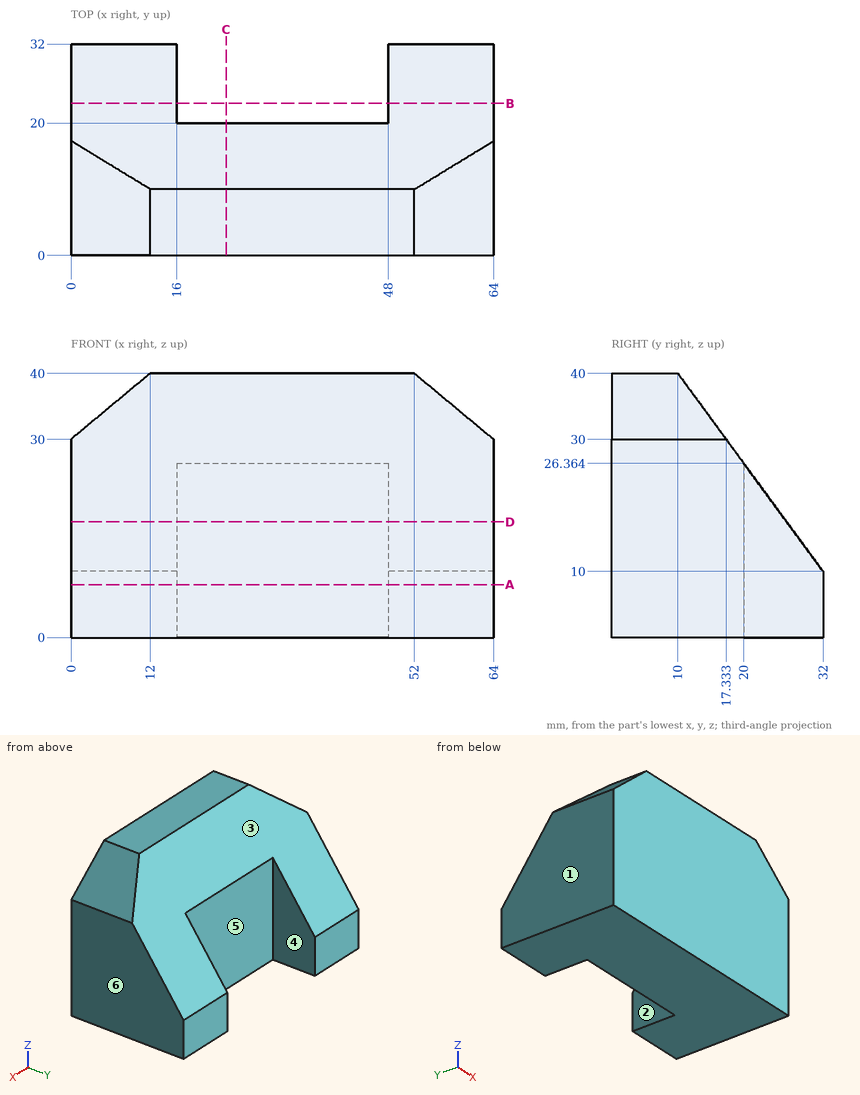
Study the drawing (mm; zero at the part's minimum x, y, z) and answer. A direction names the side the tool comes from. Coordinates: 2 decimals unless noted, no trailing zeros. Write each loop counter-clockwise with the first axis right and the second up, starting at its lowest first coordinate (ties: lowest second). Pieces come first, ordered by that corner, then holes.
Q1. Which of the six approach directions +Z, -Z, +X, -X, +Y, -Y give full straight-line access (tool end or side, diameter ignored) to the marked faces 1 and 2?
Q2. A cutting plane is placed at B-B, the plane y = 23. Give the vertices of the cut face in (x, z), then the cut area to 3 significant figures.
Q3. A cutting plane is placed at C-C, the plane x = 23.5. Give the vertices of the cut face in (y, z).
Q4. Each of these flat-tipped pins is pushed along its axis until it touches: pin 1 Ø2 at (x, z) = (24.5, 14) entering from +Y; pin 2 Ø3 at (y, z) = (14, 36) entering from +X; pin 3 Ø4 at (x, z) = (11, 13) entering from +Y. Where does it stop, or does it pass through?
Q5. A cutting plane is placed at A-A, the plane z = 8. Give the vertices of the cut face in (x, y).
Q6. Determine the mould class of the marked faces 3, 4, 5 and 6 for opening direction X: released by +X, released by -X, zero draft, split by the parting line, or undercut.
Q7. A cutting plane is placed at D-D, the plane z = 17.5. Give the vertices of the cut face in (x, y), then the cut area to 3 significant figures.
Q8. Find the intervals of material crossed by line 1 (X direction, y = 27, z = 12.5); line 2 (Y direction, x = 33, z = 6.5); line 3 (Z direction, x = 6.5, y = 6) (1 decimal), in increasing order.
Findings below:
1. face 1: +Z, -Z, -X, +Y, -Y
1. face 2: +Z, -Z, +Y
2. outline: (0, 0) - (16, 0) - (16, 22.27) - (0, 22.27) - close; (48, 0) - (64, 0) - (64, 22.27) - (48, 22.27) - close
2. area: 713 mm2
3. outline: (0, 0) - (20, 0) - (20, 26.36) - (10, 40) - (0, 40) - close
4. pin 1: stops at y = 20
4. pin 2: stops at x = 58.6
4. pin 3: stops at y = 31.27
5. outline: (0, 0) - (64, 0) - (64, 32) - (48, 32) - (48, 20) - (16, 20) - (16, 32) - (0, 32) - close
6. face 3: zero draft
6. face 4: undercut
6. face 5: undercut
6. face 6: released by +X
7. outline: (0, 0) - (64, 0) - (64, 26.5) - (48, 26.5) - (48, 20) - (16, 20) - (16, 26.5) - (0, 26.5) - close
7. area: 1,490 mm2
8. line 1: x = 0 to 16, 48 to 64
8. line 2: y = 0 to 20
8. line 3: z = 0 to 35.4
